Geometry: final body of the model. Coordinates: model frame, mm. A direction names the side the tool comes from. Give positions to 0.01 mm unless a question says otherwise; leave off trailing zeros. Order: outer loops, then holes, each group sorted by start corner. A loop starts at its lowest first (then second) coordinate and runs counter-clockwise, first axis right, second up. Notation, with made-up numbers: (-27.5, 56) - (-7.5, 56) arc R14 ccw to (-7.5, 73) - close; hole circle Ø8 at (-0.5, 84.5). An arc over 180 degrees is marked (long way). Write item = value, one per line. Start each with the question number.
from build123d import *

# Parameters (mm, degrees)
IZIM2_R                     = 3
Y_KSEKLIK_EKSTR_ZYON1_DEPTH = 6
IZIM3_R                     = 1.5
KES_EKSTR_ZYON1_DEPTH       = 3
Y_KSEKLIK_EKSTR_ZYON2_DEPTH = 29


with BuildPart() as part:
    # Çizim2 → Yükseklik-Ekstrüzyon1 (new body)
    with BuildSketch(Plane(origin=(0, 0, 0), x_dir=(1, 0, 0), z_dir=(0, 1, 0))):
        with Locations(Location((0, 0, 0), (0, 0, 270))):
            Circle(IZIM2_R)
    extrude(amount=Y_KSEKLIK_EKSTR_ZYON1_DEPTH)

    # Çizim3 → Kes-Ekstrüzyon1 (cut)
    with BuildSketch(Plane(origin=(0, 6, 0), x_dir=(1, 0, 0), z_dir=(0, 1, 0))):
        with Locations(Location((0, 0, 0), (0, 0, 270))):
            Circle(IZIM3_R)
    extrude(amount=-KES_EKSTR_ZYON1_DEPTH, mode=Mode.SUBTRACT)

    # Çizim4 → Yükseklik-Ekstrüzyon2 (add)
    with BuildSketch(Plane.XZ):
        with BuildLine():
            ThreePointArc((1.79891634, 2.08), (0, 2.75), (-1.79891634, 2.08))
            Line((-1.79891634, 2.08), (-1.79891634, -2.08))
            ThreePointArc((-1.79891634, -2.08), (0, -2.75), (1.79891634, -2.08))
            Line((1.79891634, -2.08), (1.79891634, 2.08))
        make_face()
    extrude(amount=Y_KSEKLIK_EKSTR_ZYON2_DEPTH)


solid = part.part
Q1. Contact query for flat-ended pins moving along their axis: pin 1 (1.2 mm diameter, centred on y = -18, z = 0, fed in from -X); pin 2 (3 mm diameter, centred on x = 0.5, y = -10.5, fed in from -Z); pin 3 (0.9 mm diameter, centred on x = -0.5, z = -0.5, fed in from +Y). Output: stop coordinate, or through.
Q2. Section A-A, the plane z = 0. Return the cut outline in (x, y), then the cut area to 3 significant figures.
Q3. Set-up query: faces 5 (the cylindrical face through (0.9, 2.96, 2.86)), 6 (the cylindrical face through (-0.03, -14.3, -2.75)), 7 (the flat face through (0, -29, 0)), 8 (the flat face through (-1.799, -14, 0)), 9 (the flat face through (1.799, -14, 0)). Return all of +Z, -Z, +X, -X, +Y, -Y with unobstructed straight access to the full face (end or side cutting, diameter ignored); none if empty.
Q4. Section B-B, the plane y = 3.5. Return the cut outline in (x, z).
Q5. Section C-C, the plane x = -0.4. Return the cut outline in (y, z).
Q6. Pull-direction query (Z, two-part tool) for faces 1 (the flat face through (-1.3, 6, 1.3)), 2 (the cylindrical face through (0.03, -14.3, 2.75)), 3 (the flat face through (0, 3, 0)), 4 (the cylindrical face through (0.45, 4.52, 1.43)); classes: +Z half, -Z half, draft (parallel to the pull), parting line (faces both ways), or undercut.
Q7. Material intervals for line 1 along X through (y, z) = (3.9, 0); line 2 along X through (y, z) = (-14, -1.95); line 3 along Y through (x, z) = (-1.25, -2.6), sorted ascending. Write a range as from..to.
Q8. Section D-D, the plane y = -10.5. Return the cut outline in (x, z), then the cut area to 3 significant figures.
The answers:
q1.pin_1 = -1.8
q1.pin_2 = -2.75
q1.pin_3 = 3
q2.outline = (-3, 0) - (-1.8, 0) - (-1.8, -29) - (1.8, -29) - (1.8, 0) - (3, 0) - (3, 6) - (1.5, 6) - (1.5, 3) - (-1.5, 3) - (-1.5, 6) - (-3, 6) - close
q2.area = 131 mm²
q3.face_5 = +Y, -Y
q3.face_6 = -Z, -Y
q3.face_7 = +Z, -Z, +X, -X, -Y
q3.face_8 = +Z, -Z, -X, -Y
q3.face_9 = +Z, -Z, +X, -Y
q4.outline = circle Ø6 at (0, 0); hole circle Ø3 at (0, 0)
q5.outline = (-29, -2.72) - (0, -2.72) - (0, -2.97) - (6, -2.97) - (6, -1.45) - (3, -1.45) - (3, 1.45) - (6, 1.45) - (6, 2.97) - (0, 2.97) - (0, 2.72) - (-29, 2.72) - close
q6.face_1 = draft
q6.face_2 = +Z half
q6.face_3 = undercut
q6.face_4 = undercut
q7.line_1 = -3..-1.5, 1.5..3
q7.line_2 = -1.8..1.8
q7.line_3 = 0..6
q8.outline = (-1.8, -2.08) arc R2.75 ccw to (1.8, -2.08) - (1.8, 2.08) arc R2.75 ccw to (-1.8, 2.08) - close
q8.area = 18.3 mm²
